Build history of the part. All positions in model axes, mm. Give positions to 0.01 mm unless a question says otherwise; leave off trailing zeros. Loops run counter-clockwise (first coordinate to the right, second up) from the corner with the lowest first, then second, coordinate; pieces in that order, holes last.
1) Band-saw the part on A-A on y = 1. List the corners of the cut face in (x, z), then the cut area to 3 significant figures.
2) Flat gauge pins, fed straight in: P1, Ø1.5, axis at x = 20, y = 12.5, coming from the +Z side; P2, Ø1.5, axis at x = 38.5, z = -19, coming from the +Y side; P3, Ø12, axis at y = -14.5, z = -5.5, coming from the +X side. Where does each tip first touch, or does it go through?
3) Wall check: line 1 (X direction, y = -6.5, z = -18.5); line 2 (Y direction, x = 41.5, z = -12); line 3 (Z direction, x = 40, y = -9). Give the ranges that are in metal, low to high.
4) Band-saw the part on B-B on x = 44.5. List the corners of the cut face in (y, z).
5) Band-saw the part on C-C on z = -22.5. List the corners of the cut face in (x, y), then the cut area to 3 significant figures.
Autodesk Inventor part; units mm, degrees
ref_plane "工作平面1" through (10, 22, 0) normal (-0.4795, -0.6205, -0.6205) x (0.7913, 0, -0.6114)
ref_plane "YZ Plane" through (0, 0, 0) normal (1, 0, 0) x (0, 1, 0)
ref_plane "XZ Plane" through (0, 0, 0) normal (0, 1, 0) x (-1, 0, 0)
sketch "草圖1" plane through (0, 0, 0) normal (0, 1, 0) x (-1, 0, 0)
  line L0 (0, 0) -> (-54, 0)
  line L1 (-54, 0) -> (-54, -44)
  line L2 (-54, -44) -> (0, -44)
  line L3 (0, -44) -> (0, 0)
  dimension "d0" = 54
  dimension "d1" = 44
extrude "擠出1" add sketch "草圖1" along normal mid plane 44
sketch "草圖2" plane through (0, 22, 0) normal (0, 1, 0) x (1, 0, 0)
  line L0 (0, 0) -> (54, 0)
  line L1 (10, 0) -> (54, 14)
  line L2 (54, 0) -> (54, 44)
  dimension "d4" = 10
  dimension "d5" = 30
extrude "擠出2" cut sketch "草圖2" against normal blind 60
sketch "草圖3" plane through (54, -22, -44) normal (1, 0, 0) x (0, 0, -1)
  line L0 (-30, 24) -> (-10, 44)
  line L1 (0, 44) -> (-44, 44)
  line L2 (-30, 44) -> (-30, 0)
  point P0 (-44, 22)
  point P1 (-30, 2)
  dimension "d8" = 20
  dimension "d9" = 20
ref_plane "工作平面1" through (10, 22, 0) normal (-0.4795, -0.6205, -0.6205) x (0.7913, 0, -0.6114)
sketch "草圖4" plane through (10, 22, 0) normal (-0.4795, -0.6205, -0.6205) x (0.7913, 0, -0.6114)
  line L0 (-15.1543, -12.3218) -> (93.717, -12.3218)
  line L1 (93.717, -12.3218) -> (93.717, 28.8166)
  line L2 (93.717, 28.8166) -> (-15.1543, 28.8166)
  line L3 (-15.1543, 28.8166) -> (-15.1543, -12.3218)
  point P0 (-7.9129, 13.4581)
extrude "擠出3" cut sketch "草圖4" against normal blind 40
mirror "鏡射1" about plane through (0, 0, 0) normal (0, 1, 0) of "擠出3"
properties part number "61"
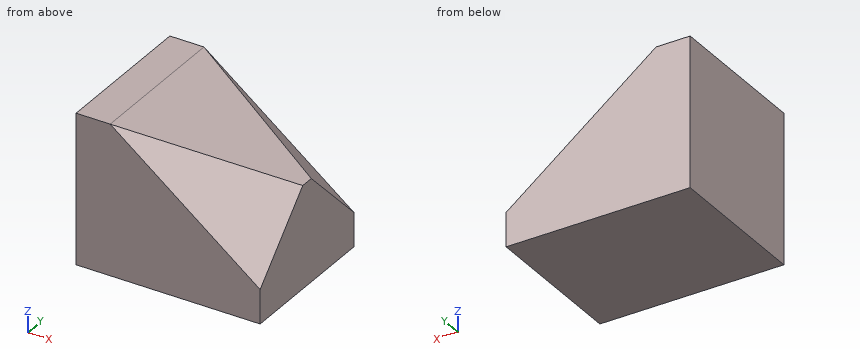
Findings below:
1. outline: (0, -44) - (54, -44) - (54, -14) - (10, 0) - (0, 0) - close
1. area: 2,070 mm2
2. P1: stops at z = -2.94
2. P2: stops at y = 19.92
2. P3: stops at x = 37.8
3. line 1: x = 0 to 53.99
3. line 2: y = -9.65 to 9.65
3. line 3: z = -44 to -10.19
4. outline: (-22, -44) - (22, -44) - (22, -26.66) - (6.31, -10.98) - (-6.31, -10.98) - (-22, -26.66) - close
5. outline: (0, -22) - (39.11, -22) - (54, -10.5) - (54, 10.5) - (39.11, 22) - (0, 22) - close
5. area: 2,200 mm2
